Source: CAD feature listing. Evaluate the final solid. Frame: model axes, mm. A direction names the side the tool comes from. Round coordinates to 2 decimals unless told otherwise and drop trailing zeros. Order: outer loops, then holes, each group sorted by start corner. A loop starts at its lowest first (then second) coordinate and runs counter-clockwise, first axis right, second up.
```python
from build123d import *

# Parameters (mm, degrees)
SKETCH1_W           = 50
SKETCH1_H           = 20
BOSS_EXTRUDE1_DEPTH = 1
BOSS_EXTRUDE2_DEPTH = 6
SKETCH3_W           = 46
SKETCH3_H           = 1
BOSS_EXTRUDE3_DEPTH = 4
SKETCH4_W           = 6.5
SKETCH4_H           = 2
SKETCH4_H_2         = 2.438820915
BOSS_EXTRUDE4_DEPTH = 6
SKETCH5_W           = 6.5
SKETCH5_H           = 1
BOSS_EXTRUDE5_DEPTH = 1.5
SKETCH6_W           = 6.5
SKETCH6_H           = 1
BOSS_EXTRUDE6_DEPTH = 1.5
CHAMFER1_SIZE       = 1.5
FILLET1_R           = 2
FILLET2_R           = 1
SKETCH7_W           = 5
SKETCH7_H           = 3.5
CUT_EXTRUDE1_DEPTH  = 2
FILLET3_R           = 2


with BuildPart() as part:
    # Sketch1 → Boss-Extrude1 (new body)
    with BuildSketch(Plane.XY):
        Rectangle(SKETCH1_W, SKETCH1_H)
    extrude(amount=BOSS_EXTRUDE1_DEPTH)

    # Sketch2 → Boss-Extrude2 (add)
    with BuildSketch(Plane.XY.offset(1)):
        Polygon((-25, 10), (25, 10), (25, 9), (25, -10), (23, -10), (23, 9), (-23, 9), (-23, -10), (-25, -10), (-25, 9), align=None)
    extrude(amount=BOSS_EXTRUDE2_DEPTH)

    # Sketch3 → Boss-Extrude3 (add)
    with BuildSketch(Plane.XZ.offset(-9)):
        with Locations((0, 6.5)):
            Rectangle(SKETCH3_W, SKETCH3_H)
    extrude(amount=BOSS_EXTRUDE3_DEPTH)

    # Sketch4 → Boss-Extrude4 (add)
    with BuildSketch(Plane.XY.offset(1)):
        with Locations((-19.75, -9)):
            Rectangle(SKETCH4_W, SKETCH4_H)
        with Locations((19.75, -8.780589542)):
            Rectangle(SKETCH4_W, SKETCH4_H_2)
    extrude(amount=BOSS_EXTRUDE4_DEPTH)

    # Sketch5 → Boss-Extrude5 (add)
    with BuildSketch(Plane(origin=(0, -8, 0), x_dir=(1, 0, 0), z_dir=(0, 1, 0))):
        with Locations((-19.75, -6.5)):
            Rectangle(SKETCH5_W, SKETCH5_H)
    extrude(amount=BOSS_EXTRUDE5_DEPTH)

    # Sketch6 → Boss-Extrude6 (add)
    with BuildSketch(Plane(origin=(0, -7.561179085, 0), x_dir=(1, 0, 0), z_dir=(0, 1, 0))):
        with Locations((19.75, -6.5)):
            Rectangle(SKETCH6_W, SKETCH6_H)
    extrude(amount=BOSS_EXTRUDE6_DEPTH)

    # Chamfer1
    chamfer1_edges = [part.edges().sort_by_distance(p)[0] for p in [
        (16.5, -6.061179085, 6.5),
        (-16.5, -6.5, 6.5),
    ]]
    chamfer(chamfer1_edges, length=CHAMFER1_SIZE)

    # Fillet1
    fillet1_edges = [part.edges().sort_by_distance(p)[0] for p in [
        (25, -10, 3.5),
        (-25, -10, 3.5),
        (-25, 10, 3.5),
        (25, 10, 3.5),
    ]]
    fillet(fillet1_edges, radius=FILLET1_R)

    # Fillet2
    fillet2_edges = [part.edges().sort_by_distance(p)[0] for p in [
        (23, 9, 3.5),
        (-23, 9, 3.5),
        (-23, -8, 3.5),
        (23, -7.561179085, 3.5),
    ]]
    fillet(fillet2_edges, radius=FILLET2_R)

    # Sketch7 → Cut-Extrude1 (cut)
    with BuildSketch(Plane.XY.offset(7)):
        with Locations((0, 6.75)):
            Rectangle(SKETCH7_W, SKETCH7_H)
    extrude(amount=-CUT_EXTRUDE1_DEPTH, mode=Mode.SUBTRACT)

    # Fillet3
    fillet3_edges = [part.edges().sort_by_distance(p)[0] for p in [
        (-2.5, 5, 6.5),
        (2.5, 5, 6.5),
    ]]
    fillet(fillet3_edges, radius=FILLET3_R)


solid = part.part
```
1. Section D-D on x = -3. Return loops of the section in (y, z), plus the area to 3 significant figures.
2. Section B-B on y = 4. Return loops of the section in (x, z), plus the area to 3 significant figures.
3. Line query: line 1 along X through (y, z) = (-3, 6.25); line 2 along Y through (x, z) = (17, 3.5); line 3 along Z through (x, y) = (-8, 7.5). Output: solid intervals per line, ascending.
4. Section A-A on x = 17.5. Return loops of the section in (y, z), plus the area to 3 significant figures.
5. Section C-C on z = 2.75. Return loops of the section in (x, y).
6. Access query for faces 5 (the face through (19, -7.561, 3)), 6 (the face through (-17.3, -7.2, 6.5)), 7 (the face through (3.1, 5.57, 6.49)). Directions: +Z, -Z, +X, -X, +Y, -Y. A direction counts if a zero-diameter tool reaches every point of the face in a straight line with its end or side. Return the directions, or none.
7. First-contact query: pin 1 (0.5 mm diameter, centred on x = -13, z = 6.5, fed in from -Y); pin 2 (4 mm diameter, centred on x = -12.5, y = -4.5, fed in from +Z); pin 3 (1.1 mm diameter, centred on x = 0, z = 6.5, fed in from -Y). Flat tips, straight axial feed; report the tip coordinate or a pass-through.
8. Pull-direction query (X, two-part tool) for faces 1 (the face through (-16.5, -9, 4)), 2 (the face through (25, 0, 3)), 3 (the face through (0, 0, 0)), 4 (the face through (-24.4, 9.43, 3.55)); classes: released by +X, released by -X, zero draft, split by the parting line, or undercut.
Result:
1. outline: (-10, 0) - (10, 0) - (10, 7) - (5.68, 7) - (5.68, 6) - (9, 6) - (9, 1) - (-10, 1) - close
1. area: 29.3 mm2
2. outline: (-25, 0) - (25, 0) - (25, 7) - (23, 7) - (23, 1) - (-23, 1) - (-23, 7) - (-25, 7) - close
2. area: 74.0 mm2
3. line 1: x = -25 to -23, 23 to 25
3. line 2: y = -10 to -7.56, 9 to 10
3. line 3: z = 0 to 1, 6 to 7
4. outline: (-10, 0) - (10, 0) - (10, 7) - (5, 7) - (5, 6) - (9, 6) - (9, 1) - (-7.56, 1) - (-7.56, 6) - (-6.56, 6) - (-6.56, 7) - (-10, 7) - close
4. area: 45.6 mm2
5. outline: (-25, -8) arc R2 ccw to (-23, -10) - (-16.5, -10) - (-16.5, -8) - (-22, -8) arc R1 cw to (-23, -7) - (-23, 8) arc R1 cw to (-22, 9) - (22, 9) arc R1 cw to (23, 8) - (23, -6.56) arc R1 cw to (22, -7.56) - (16.5, -7.56) - (16.5, -10) - (23, -10) arc R2 ccw to (25, -8) - (25, 8) arc R2 ccw to (23, 10) - (-23, 10) arc R2 ccw to (-25, 8) - close
6. face 5: none
6. face 6: +Z
6. face 7: +Z, -Y
7. pin 1: stops at y = 5
7. pin 2: stops at z = 1
7. pin 3: stops at y = 8.5
8. face 1: undercut
8. face 2: released by +X
8. face 3: zero draft
8. face 4: released by -X
